Design review of the part built by this model. Coordinates are the model's own, in mm. Face numbers are marked on the shaded views. Round coordinates to 2 decimals unless told otherwise and drop trailing zeros. Order: outer loops, then holes, each group sorted by start corner. A loop starts at its lowest first (then second) coordinate and runs counter-clockwise, first axis right, second up.
from build123d import *

# Parameters (mm, degrees)
SCHIZZO1_W                   = 100
SCHIZZO1_H                   = 100
SCHIZZO1_R                   = 6
ESTRUSIONE_ESTRUSIONE1_DEPTH = 10
RACCORDO1_R                  = 10


with BuildPart() as part:
    # Schizzo1 → Estrusione-Estrusione1 (new body)
    with BuildSketch(Plane(origin=(0, 0, 0), x_dir=(1, 0, 0), z_dir=(0, 1, 0))):
        Rectangle(SCHIZZO1_W, SCHIZZO1_H)
        with Locations(Location((-35, 35, 0), (0, 0, 270))):
            Circle(SCHIZZO1_R, mode=Mode.SUBTRACT)
        with Locations(Location((35, 35, 0), (0, 0, 270))):
            Circle(SCHIZZO1_R, mode=Mode.SUBTRACT)
        with Locations(Location((-35, -35, 0), (0, 0, 270))):
            Circle(SCHIZZO1_R, mode=Mode.SUBTRACT)
        with Locations(Location((35, -35, 0), (0, 0, 270))):
            Circle(SCHIZZO1_R, mode=Mode.SUBTRACT)
    extrude(amount=ESTRUSIONE_ESTRUSIONE1_DEPTH)

    # Raccordo1
    raccordo1_edges = [part.edges().sort_by_distance(p)[0] for p in [
        (-50, 5, -50),
        (50, 5, -50),
        (50, 5, 50),
        (-50, 5, 50),
    ]]
    fillet(raccordo1_edges, radius=RACCORDO1_R)


solid = part.part
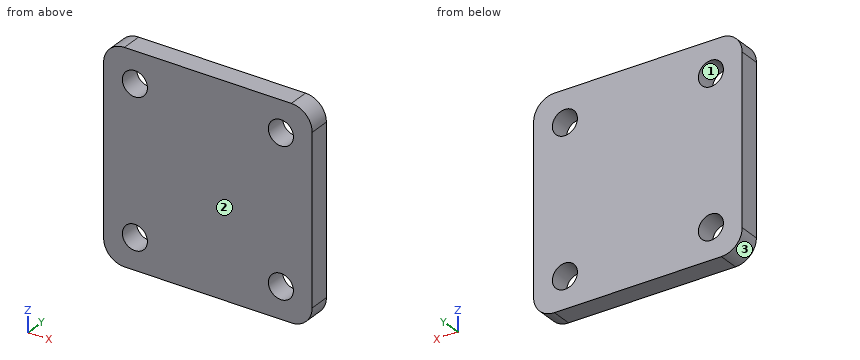
1) Take a section at A-A on z = -35. Give the boundary of the cut face in (x, y), plus the area to 3 significant figures.
Results:
outline: (-50, 0) - (-41, 0) - (-41, 10) - (-50, 10) - close; (-29, 0) - (29, 0) - (29, 10) - (-29, 10) - close; (41, 0) - (50, 0) - (50, 10) - (41, 10) - close
area: 760 mm2
2) Clearance check with a flat-ended pin moving along its axis: P1, Ø19, axis at x = 35, z = 35, coming from the -Y side. State where the tip first meets the part, or that it passes through.
Results:
P1: stops at y = 0
3) The part is to be moulded in two halves that separate along X. For the marked faces 1, 2 and 3, say which applies: released by +X, released by -X, zero draft, split by the parting line, or undercut.
Results:
face 1: undercut
face 2: zero draft
face 3: released by -X
4) Take a section at C-C on y = 3.75. Give the boundary of the cut face in (x, z), plus the area to 3 significant figures.
Results:
outline: (-50, -40) arc R10 ccw to (-40, -50) - (40, -50) arc R10 ccw to (50, -40) - (50, 40) arc R10 ccw to (40, 50) - (-40, 50) arc R10 ccw to (-50, 40) - close; hole circle Ø12 at (-35, -35); hole circle Ø12 at (-35, 35); hole circle Ø12 at (35, -35); hole circle Ø12 at (35, 35)
area: 9,460 mm2
5) Take a section at B-B on x = 35. Give the boundary of the cut face in (y, z), plus the area to 3 significant figures.
Results:
outline: (0, -50) - (10, -50) - (10, -41) - (0, -41) - close; (0, -29) - (10, -29) - (10, 29) - (0, 29) - close; (0, 41) - (10, 41) - (10, 50) - (0, 50) - close
area: 760 mm2
6) To check wall thickness, follow line 1 along X through (y, z) = (3.25, -35); line 2 along X through (y, z) = (1.5, -29.5); line 3 along Z through (x, y) = (30.5, 5). State the ranges of each line that lie inside material, in increasing order.
Results:
line 1: x = -50 to -41, -29 to 29, 41 to 50
line 2: x = -50 to -37.4, -32.6 to 32.6, 37.4 to 50
line 3: z = -50 to -38.97, -31.03 to 31.03, 38.97 to 50
